CAD build for the part. Positions are in the model's coordinates, mm. A direction names the side the tool comes from. Give positions to 0.01 mm unless a question says otherwise; leave off trailing zeros. Order: outer loops, then holes, each group sorted by start corner. A loop starts at its lowest first (then second) coordinate and runs counter-clockwise, first axis right, second up.
```python
from build123d import *

# Parameters (mm, degrees)
F0_W     = 43.18
F0_H     = 5.932273
F0_W_2   = 5.932274
F0_H_2   = 58.42
F1_DEPTH = 11.938


with BuildPart() as f1:
    # F0 (on Top) → F1 (new body)
    with BuildSketch(Plane.XY):
        with Locations((-6.381456, 6.09027)):
            Rectangle(F0_W, F0_H)
        with BuildLine():
            Line((-27.971456, 3.124134), (-27.971456, 9.056407))
            Line((-27.971456, 9.056407), (-33.90373, 9.056407))
            ThreePointArc((-33.90373, 9.056407), (-32.166207, 4.861656), (-27.971456, 3.124134))
        make_face()
        with Locations((-30.937593, 38.266407)):
            Rectangle(F0_W_2, F0_H_2)
        with BuildLine():
            Line((21.140817, 9.056407), (15.208544, 9.056407))
            Line((15.208544, 9.056407), (15.208544, 3.124134))
            ThreePointArc((15.208544, 3.124134), (19.403295, 4.861656), (21.140817, 9.056407))
        make_face()
        Polygon((15.208544, 67.476407), (15.208544, 9.056407), (21.140817, 9.056407), (21.152144, 9.056407), (21.152144, 67.476407), align=None)
    extrude(amount=F1_DEPTH)


solid = f1.part
```
Item 1: Slice it at A-A (y = 54). Give the cut face in (x, z).
Item 2: Slice it at C-C (x = -11). Give the cut face in (y, z).
Item 3: Two-plate mould, pull along X, no slides. Class faces 1 (the face through (19.36, 4.82, 5.89)), 2 (the face through (15.209, 39, 6)), 3 (the face through (-32.212, 4.908, 5.885)), 4 (the face through (-7, 9.056, 6)): released by +X, released by -X, zero draft, split by the parting line, or undercut.
Item 4: Wall check: L1, parallel to X at y = 28, z = 2; L2, parallel to Y at x = -27.5, z = 4.25; L3, parallel to Y at x = 18.5, z = 10.75. Give the ranges that are in metal, low to high.
Item 5: Tool access for faces 5 (the face through (-7, 3.124, 6)), 6 (the face through (-27.971, 38, 6)): list every direction of +Z, -Z, +X, -X, +Y, -Y with a clear straight run to the whole face (end or side of a thin tool).
A:
1. outline: (-33.9, 0) - (-27.97, 0) - (-27.97, 11.94) - (-33.9, 11.94) - close; (15.21, 0) - (21.15, 0) - (21.15, 11.94) - (15.21, 11.94) - close
2. outline: (3.12, 0) - (9.06, 0) - (9.06, 11.94) - (3.12, 11.94) - close
3. face 1: released by +X
3. face 2: undercut
3. face 3: released by -X
3. face 4: undercut
4. L1: x = -33.9 to -27.97, 15.21 to 21.15
4. L2: y = 3.12 to 9.06
4. L3: y = 4.12 to 67.48
5. face 5: +Z, -Z, +X, -X, -Y
5. face 6: +Z, -Z, +Y
